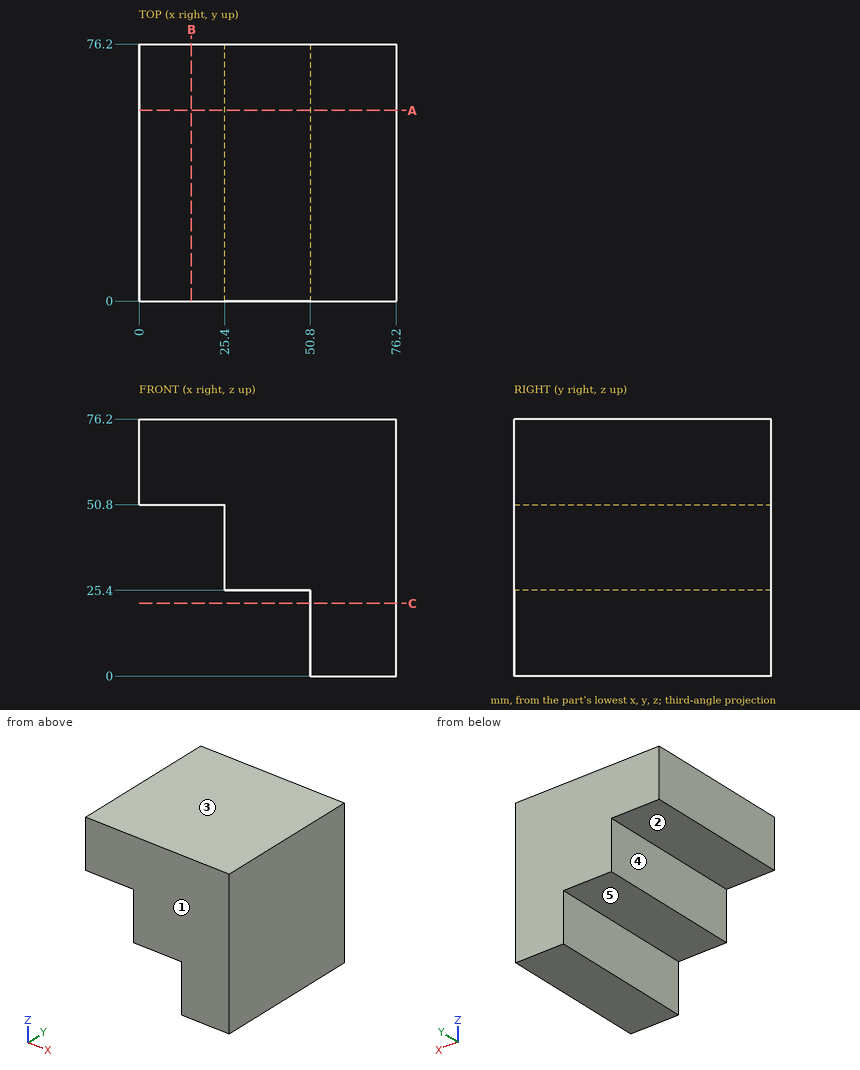
Answer from the drawing. Dimensions are ordinates in mm from the lowest x, y and z of the part. A direction names the side the tool comes from. Give positions to 0.01 mm unless a question says otherwise; leave off trailing zeros. Loops run counter-clockwise (first coordinate to the right, second up) from the corner with the lowest first, then second, coordinate; pieces in that order, holes last. Notation, with made-up numbers: M -34,-39.5 L -3,-39.5 A15 cw -3,-18.5 Z; hole C 36.5,-23 d1. An arc over 180 degrees is marked long. One line per item, written item: value.
Q1. A cutting plane is placed at C-C on z = 21.5. Determine the outline of the cut face in (x, y), then the cut area to 3 significant figures.
Working result:
outline: M 50.8,0 L 76.2,0 L 76.2,76.2 L 50.8,76.2 Z
area: 1,940 mm^2
Q2. Find the intervals of material crossed by line 1 (Z direction, x = 31.5, y = 7.5); line 2 (Z direction, x = 6, y = 66), in increasing order. Write a range as from..to.
Working result:
line 1: z = 25.4..76.2
line 2: z = 50.8..76.2
Q3. A cutting plane is placed at A-A on y = 56.5. Determine the outline of the cut face in (x, z), then the cut area to 3 significant figures.
Working result:
outline: M 0,50.8 L 25.4,50.8 L 25.4,25.4 L 50.8,25.4 L 50.8,0 L 76.2,0 L 76.2,76.2 L 0,76.2 Z
area: 3,870 mm^2
Q4. A cutting plane is placed at B-B on x = 15.5. Determine the outline of the cut face in (y, z), then the cut area to 3 significant figures.
Working result:
outline: M 0,50.8 L 76.2,50.8 L 76.2,76.2 L 0,76.2 Z
area: 1,940 mm^2
Q5. Determine the mould class of the marked faces 3, 4 and 5 for opening direction Z: +Z half, -Z half, draft (parallel to the pull), parting line (faces both ways), or undercut.
Working result:
face 3: +Z half
face 4: draft
face 5: -Z half
Q6. For the marked faces 1 and 2, determine the directions among +Z, -Z, +X, -X, +Y, -Y from which every point of the face is accessible in a straight line to the end or side of a thin tool.
Working result:
face 1: +Z, -Z, +X, -X, -Y
face 2: -Z, -X, +Y, -Y
Q7. Flat-ended cylindrical pins translate along their axes: P1, Ø12, axis at x = 34.5, y = 31.5, coming from the -Z side; P2, Ø1.5, axis at y = 14.5, z = 45, coming from the -X side; P3, Ø7.5, axis at y = 34, z = 9, coming from the -X side. Find the tip coordinate at first contact, or state that the pin passes through.
Working result:
P1: stops at z = 25.4
P2: stops at x = 25.4
P3: stops at x = 50.8
